CAD build for the part. Positions are in the model's coordinates, mm. A direction names the side the tool comes from. Give positions to 0.01 mm unless a question says otherwise; leave off trailing zeros. Loops run counter-clockwise (first coordinate to the right, second up) from the corner with the lowest first, then second, coordinate; pieces in that order, holes last. Notation, with made-up numbers: (-1.75, -3) -> (46.25, -3) arc R19 ccw to (46.25, 24) -> close; hole circle Ø9 at (77.5, -5). An arc over 180 degrees is marked (long way). Write each question's results on one line, items separated by ' | '. Start each with the question number.
Autodesk Inventor part; units mm, degrees
ref_plane "YZ Plane" through (0, 0, 0) normal (1, 0, 0) x (0, 1, 0)
ref_plane "XZ Plane" through (0, 0, 0) normal (0, 1, 0) x (-1, 0, 0)
ref_plane "XY Plane" through (0, 0, 0) normal (0, 0, 1) x (1, 0, 0)
sketch "Эскиз3" plane through (0, 0, 0) normal (0, 0, 1) x (1, 0, 0)
  line L0 (0, 0) -> (80, 0)
  line L1 (80, 0) -> (80, 102)
  line L2 (0, 102) -> (0, 0)
  circle A0 centre (40, 102) radius 10
  arc A1 (77.5, 102) -> (2.5, 102) centre (40, 102) ccw
  line L3 (80, 102) -> (77.5, 102)
  line L4 (2.5, 102) -> (0, 102)
  dimension "d8" = 102
  dimension "d9" = 80
  dimension "d10" = 20
  dimension "d11" = 75
extrude "Выдавливание3" add sketch "Эскиз3" along normal blind 3
equation "\"d9\" = width_coxa"
equation "\"d10\" = d_main_shaft"
equation "\"d6\" = thickness_steel"
equation "\"tolerance_plazma\" = 0.1"
equation "\"thickness_steel\" = 3"
equation "\"d_main_screw_holes\" = 6.1"
equation "\"d_main_shaft\" = 20"
equation "\"thickness_profile_tibea\" = 4"
equation "\"thickness_profile_femur\" = 3"
equation "\"width_shaft_shift\" = 35"
equation "\"width_flattened_surface\" = 12"
equation "\"width_coxa\" = 80"
properties part number "coxa_upper_steel" material "Сталь"
Q1. Saw through at A-A, the plane x = 40. List the corners of the cut face in (y, z), then the cut area to 4 significant figures.
Q2. Wall check: L1, parallel to Y at x = 40, z = 2.3; L2, parallel to Y at x = 37, z = 2.2; L3, parallel to X at y = 108.5, z = 2.6. Give the ranges that are in metal, low to high.
Q3. Drop a flat-ended pin along its axis: pin 1 (16 mm diameter, centred on x = 40, y = 102, fed in from +Z). Give the stop position or say it passes through.
Q4. Mould opens along X. For faces 1 (the face through (38.698, 92.085, 1.479)), 2 (the face through (79, 102, 1)), 3 (the face through (0, 52, 1)) say: pulls with the +X half, pulls with the -X half, needs draft (parallel to the pull), parting line crosses it, or undercut.
Q5. Saw through at C-C, the plane x = 21.5. List the corners of the cut face in (y, z).
Q6. Which spindle directions (+Z, -Z, +X, -X, +Y, -Y) get a long thin tool onto all of the face, cutting with end or side? Do faces 4 (the face through (1, 102, 1)), 5 (the face through (39, 71, 3)). Say none if no direction does.
Q7. Saw through at D-D, the plane y = 116.5. List the corners of the cut face in (x, z), then the cut area to 4 significant figures.
Q8. Saw through at B-B, the plane z = 1.4. List the corners of the cut face in (x, y), then the cut area to 3 significant figures.
Answer block:
1) outline: (0, 0) -> (92, 0) -> (92, 3) -> (0, 3) -> close; (112, 0) -> (139.5, 0) -> (139.5, 3) -> (112, 3) -> close | area: 358.5 mm2
2) L1: y = 0 to 92, 112 to 139.5 | L2: y = 0 to 92.46, 111.54 to 139.38 | L3: x = 3.07 to 32.4, 47.6 to 76.93
3) pin 1: passes through
4) face 1: undercut | face 2: needs draft | face 3: pulls with the -X half
5) outline: (0, 0) -> (134.62, 0) -> (134.62, 3) -> (0, 3) -> close
6) face 4: +Z, -Z, -X, +Y | face 5: +Z, +X, -X, +Y, -Y
7) outline: (5.42, 0) -> (74.58, 0) -> (74.58, 3) -> (5.42, 3) -> close | area: 207.5 mm2
8) outline: (0, 0) -> (80, 0) -> (80, 102) -> (77.5, 102) arc R37.5 ccw to (2.5, 102) -> (0, 102) -> close; hole circle Ø20 at (40, 102) | area: 10,100 mm2
